```python
from build123d import *

# Parameters (mm, degrees)
SKETCH1_R           = 63.5
SKETCH1_R_2         = 19.05
BOSS_EXTRUDE1_DEPTH = 12.7
SKETCH2_R           = 57.15
CUT_EXTRUDE1_DEPTH  = 6.35
SKETCH3_R           = 45
SKETCH3_R_2         = 40
BOSS_EXTRUDE3_DEPTH = 20


with BuildPart() as part:
    # Sketch1 → Boss-Extrude1 (new body)
    with BuildSketch(Plane(origin=(0, 0, 0), x_dir=(1, 0, 0), z_dir=(0, 1, 0))):
        with Locations(Location((0, 0, 0), (0, 0, 270))):
            Circle(SKETCH1_R)
        with Locations(Location((0, 0, 0), (0, 0, 270))):
            Circle(SKETCH1_R_2, mode=Mode.SUBTRACT)
    extrude(amount=BOSS_EXTRUDE1_DEPTH)

    # Sketch2 → Cut-Extrude1 (cut)
    with BuildSketch(Plane.XZ):
        with Locations(Location((0, 0, 0), (0, 0, 270))):
            Circle(SKETCH2_R)
    extrude(amount=-CUT_EXTRUDE1_DEPTH, mode=Mode.SUBTRACT)

    # Sketch3 → Boss-Extrude3 (add)
    with BuildSketch(Plane(origin=(0, 12.7, 0), x_dir=(1, 0, 0), z_dir=(0, 1, 0))):
        with Locations(Location((0, 0, 0), (0, 0, 270))):
            Circle(SKETCH3_R)
        with Locations(Location((0, 0, 0), (0, 0, 270))):
            Circle(SKETCH3_R_2, mode=Mode.SUBTRACT)
    extrude(amount=BOSS_EXTRUDE3_DEPTH)


solid = part.part
```
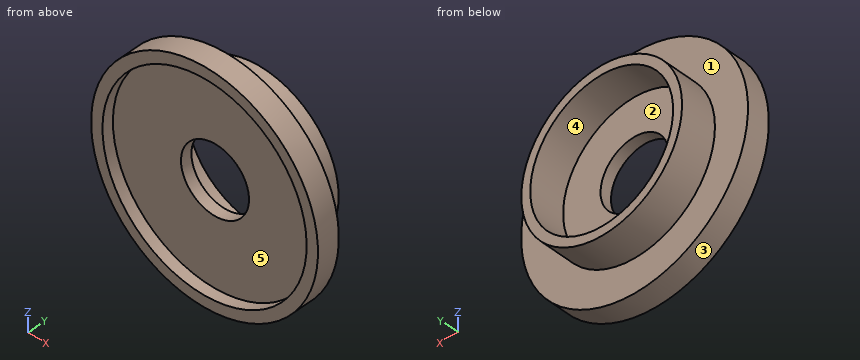
Design review of the part built by this model. Coordinates are the model's own, in mm. Face numbers are marked on the shaded views. A direction names the side the tool comes from. Give positions to 0.01 mm unless a question says otherwise; leave off trailing zeros. Loops run counter-clockwise (first coordinate to the right, second up) from the corner with the lowest first, then second, coordinate; pieces in that order, holes last. Notation, with made-up numbers: M 55.5,50.25 L 63.5,50.25 A7 ccw 63.5,59.25 Z; hole C 40.25,-12 d1. An arc over 180 degrees is marked long. Return JSON: item names as keys, results as strings. Group by question number.
Item 1: For probe 1 along X at (y, z) = (10.75, 0); probe 2 along X at (y, z) = (26, -0.5); probe 3 along Y at (x, z) = (-56.5, -13.5), list the stretches that pass through material, from the lowest coordinate up.
Item 2: We need section B-B (x = 0). Give the boundary of the cut face in (y, z), and give its area (3 significant figures).
Item 3: Tool access review of the marked faces 4 and 5: name each direction out of +Z, -Z, +X, -X, +Y, -Y from which nothing blocks a thin tool from reaching the whole face with its end or side.
Item 4: Mouldability with a two-part tool opening along X and no side actions: class the marked faces 1, 2 and 3 as released by +X, released by -X, zero draft, split by the parting line, or undercut.
Item 5: Insertion check: pin 1 Ø10 at (y, z) = (12, -14) entering from +X; pin 2 Ø4 at (x, z) = (-10.5, -11.5) entering from -Y; pin 3 Ø1 at (y, z) = (29, -12) entering from -X; pin 4 Ø1.5 at (x, z) = (-5.5, -37.5) entering from -Y. Each pin has a flat end and moves straight along its axis. Give the tip position at first contact, or say it passes through.
Item 6: We need section A-A (z = 0). Give the boundary of the cut face in (x, y).
Item 7: We need section D-D (x = 27). Give the boundary of the cut face in (y, z), and give its area (3 significant figures).
Item 8: We need section C-C (y = 8.5). Give the boundary of the cut face in (x, z).
Output:
{
 "1": {"probe 1": "x = -63.5 to -19.05, 19.05 to 63.5", "probe 2": "x = -45 to -40, 40 to 45", "probe 3": "y = 0 to 12.7"},
 "2": {"outline": "M 0,-63.5 L 12.7,-63.5 L 12.7,-45 L 32.7,-45 L 32.7,-40 L 12.7,-40 L 12.7,-19.05 L 6.35,-19.05 L 6.35,-57.15 L 0,-57.15 Z; M 0,57.15 L 6.35,57.15 L 6.35,19.05 L 12.7,19.05 L 12.7,40 L 32.7,40 L 32.7,45 L 12.7,45 L 12.7,63.5 L 0,63.5 Z", "area": "845 mm^2"},
 "3": {"face 4": "+Y", "face 5": "-Y"},
 "4": {"face 1": "zero draft", "face 2": "undercut", "face 3": "split by the parting line"},
 "5": {"pin 1": "stops at x = 62.86", "pin 2": "passes through", "pin 3": "stops at x = -43.51", "pin 4": "stops at y = 6.35"},
 "6": {"outline": "M -63.5,0 L -57.15,0 L -57.15,6.35 L -19.05,6.35 L -19.05,12.7 L -40,12.7 L -40,32.7 L -45,32.7 L -45,12.7 L -63.5,12.7 Z; M 19.05,6.35 L 57.15,6.35 L 57.15,0 L 63.5,0 L 63.5,12.7 L 45,12.7 L 45,32.7 L 40,32.7 L 40,12.7 L 19.05,12.7 Z"},
 "7": {"outline": "M 0,-57.47 L 12.7,-57.47 L 12.7,-36 L 32.7,-36 L 32.7,-29.51 L 12.7,-29.51 L 12.7,29.51 L 32.7,29.51 L 32.7,36 L 12.7,36 L 12.7,57.47 L 0,57.47 L 0,50.37 L 6.35,50.37 L 6.35,-50.37 L 0,-50.37 Z", "area": "1,080 mm^2"},
 "8": {"outline": "C 0,0 d127; hole C 0,0 d38.1"}
}
